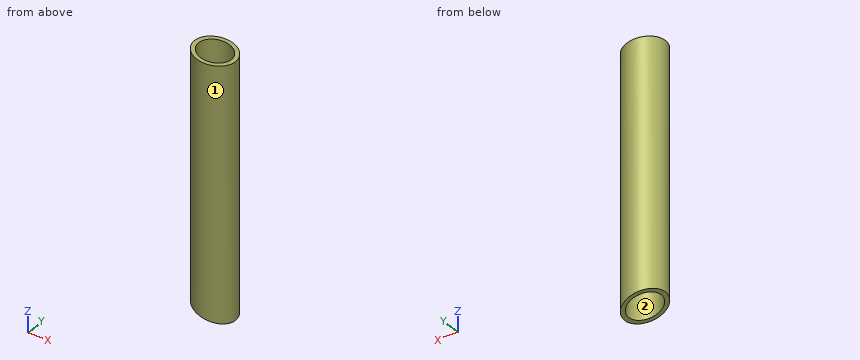
Autodesk Inventor part; units mm, degrees
ref_plane "Start plane" through (0, 0, -50.0328) normal (0, 0, 1) x (1, 0, 0)
ref_plane "End plane" through (0, 0, 160.8343) normal (0, 0, 1) x (1, 0, 0)
ref_plane "Work Plane4" through (366.1399, 0, -166.4914) normal (-0.3162, 0, -0.9487) x (-0.9487, 0, 0.3162)
ref_plane "Start plane" through (0, 0, -50.0328) normal (0, 0, 1) x (1, 0, 0)
ref_plane "End plane" through (0, 0, 160.8343) normal (0, 0, 1) x (1, 0, 0)
sketch "Sketch" plane through (0, 0, 0) normal (0, 0, 1) x (1, 0, 0)
  circle A0 centre (0, 0) radius 13.3858
  circle A1 centre (0, 0) radius 16.764
  dimension "d0" = 33.528
  dimension "d1" = 3.3782
extrude "Body" add sketch "Sketch" along normal up to surface (210.8671 mm away) from surface at -50.0328
sketch "Sketch3" plane through (0, 0, 0) normal (0, 0, 1) x (1, 0, 0)
  line L0 (0, 0) -> (10, 0)
ref_plane "Work Plane3" through (0, 0, 0) normal (0, -1, 0) x (1, 0, 0)
ref_plane "Work Plane4" through (366.1399, 0, -166.4914) normal (-0.3162, 0, -0.9487) x (-0.9487, 0, 0.3162)
split "Split1" plane through (366.1399, 0, -166.4914) removes the side toward (-0.3162, 0, -0.9487)
ref_plane "Work Plane5" through (-16.764, 0, 160.8343) normal (0.1602, 0, 0.9871) x (0.9871, 0, -0.1602)
split "Split2" plane through (-16.764, 0, 160.8343) removes the side toward (0.1602, 0, 0.9871)
sketch "Sketch4" plane through (0, 0, 0) normal (0, -1, 0) x (1, 0, 0)
  line L0 (-2, -50.0328) -> (12, -50.0328)
  line L1 (-2, 160.8343) -> (12, 160.8343)
  dimension "d7" = 210.8671
equation "\"d0\" = G_H"
equation "\"d1\" = G_T"
equation "\"d2\" = G_L"
equation "\"G_H\" = 33.528"
equation "\"G_T\" = 3.3782"
equation "\"G_L\" = d7"
equation "\"G_OFFSET_START\" = 50.03276"
equation "\"G_OFFSET_END\" = 2.72042"
equation "\"d4\" = -G_OFFSET_START"
equation "\"d5\" = G_OFFSET_END + B_L"
equation "\"B_L\" = 158.11388"
properties part number "ANSI - 1 x 0.133 - 8.302" material "Steel, Mild"
Can you work these out from the model? Positions are in its coordinate system, mm. Face numbers are marked on the shaded views. Coordinates: 2 decimals unless noted, no trailing zeros. Loops run counter-clockwise (first coordinate to the right, second up) from the corner with the lowest first, then second, coordinate; pieces in that order, holes last. Notation, with made-up numbers: M 8,80 L 28,80 A29 ccw 28,113 Z; hole C 12.5,33 d10. An arc over 180 degrees is marked long. Put each result on its own line as item: value. Start each with the question number.
(1) Imagine slicing it at A-A on x = 3. List the corners of the cut face in (y, z) for me.
(2) Imagine slicing it at B-B on y = -6. List the corners of the cut face in (x, z) for me.
(3) Imagine slicing it at C-C on z = 99. List the corners of the cut face in (x, y) for me.
(4) Will these pins go through, and if not, where does the flat tip stop? pin 1 Ø8 at (x, y) = (0.5, -12.5) entering from +Z; pin 2 Ø8 at (x, z) = (-9.5, 10.5) entering from -Y; pin 3 Ø8 at (x, y) = (10, -5) entering from +Z.
(5) We'd pull the mould along X, two halves only. Please class the marked faces 1 and 2: +X half, -X half, draft (parallel to the pull), parting line (faces both ways), or undercut.
(6) I need wall thicknesses on probe 1 along Y at (x, z) = (0, 16); probe 2 along Y at (x, z) = (-1, -20). Which ranges of each line are inside material? Lowest first, please.
Worked answers:
1. outline: M -16.49,-45.46 L -13.05,-45.46 L -13.05,157.63 L -16.49,157.63 Z; M 13.05,-45.46 L 16.49,-45.46 L 16.49,157.63 L 13.05,157.63 Z
2. outline: M -15.65,-39.24 L -11.97,-40.47 L -11.97,160.06 L -15.65,160.65 Z; M 11.97,-48.45 L 15.65,-49.67 L 15.65,155.57 L 11.97,156.17 Z
3. outline: C 0,0 d33.53; hole C 0,0 d26.77
4. pin 1: stops at z = 158.68
4. pin 2: stops at y = -15.84
4. pin 3: stops at z = 156.51
5. face 1: parting line
5. face 2: undercut
6. probe 1: y = -16.76 to -13.39, 13.39 to 16.76
6. probe 2: y = -16.73 to -13.35, 13.35 to 16.73
